Input: part model. Units: mm. Frame: model coordinates. A direction names the side the tool comes from. Coordinates: 2 decimals unless noted, no trailing zeros. Write each loop counter-clockwise with the first axis right and the second up, starting at its lowest first coordinate (ties: lowest second). Pieces come first, ordered by that corner, then holes. Notation, with made-up numbers: M 73.5,-15 L 117.5,-15 A14 cw 117.5,3 Z; hole C 34,64.5 d4. An arc over 180 degrees is marked long. Use one line per item in the form item = value.
from build123d import *

# Parameters (mm, degrees)
BOSS_EXTRUDE1_DEPTH = 60
SKETCH2_R           = 1.55
CUT_EXTRUDE1_DEPTH  = 6
SKETCH4_W           = 35
SKETCH4_H           = 30
CUT_EXTRUDE3_DEPTH  = 15
SKETCH5_R           = 1.35
CUT_EXTRUDE4_DEPTH  = 5


with BuildPart() as part:
    # Sketch1 → Boss-Extrude1 (new body)
    with BuildSketch(Plane(origin=(0, 0, 0), x_dir=(1, 0, 0), z_dir=(0, 1, 0))):
        with BuildLine():
            ThreePointArc((-42.142615011, 25), (-48.692157925, 5.483954466), (-46.647615159, -15))
            Line((-46.647615159, -15), (-41.36423576, -15))
            Line((-41.36423576, -15), (-35, -15))
            Line((-35, -15), (-35, -10))
            Line((-35, -10), (-42.848570571, -10))
            ThreePointArc((-42.848570571, -10), (-43.67673377, 5.323807579), (-39.191835885, 20))
            Line((-39.191835885, 20), (-35, 20))
            Line((-35, 20), (-35, 25))
            Line((-35, 25), (-36.20773398, 25))
            Line((-36.20773398, 25), (-42.142615011, 25))
        make_face()
    extrude(amount=BOSS_EXTRUDE1_DEPTH)

    # Sketch2 → Cut-Extrude1 (cut, through all)
    with BuildSketch(Plane(origin=(0, 0, 10), x_dir=(-1, 0, 0), z_dir=(0, 0, -1))):
        with Locations((39.997615159, 50)):
            Circle(SKETCH2_R)
        with Locations((39.997615159, 10)):
            Circle(SKETCH2_R)
    extrude(amount=-CUT_EXTRUDE1_DEPTH, mode=Mode.SUBTRACT)

    # Sketch4 → Cut-Extrude3 (cut, through all)
    with BuildSketch(Plane(origin=(-35, 0, 0), x_dir=(0, 0, -1), z_dir=(1, 0, 0))):
        with Locations((7.5, 30)):
            Rectangle(SKETCH4_W, SKETCH4_H)
    extrude(amount=-CUT_EXTRUDE3_DEPTH, mode=Mode.SUBTRACT)

    # Sketch5 → Cut-Extrude4 (cut)
    with BuildSketch(Plane(origin=(-35, 0, 0), x_dir=(0, 0, -1), z_dir=(1, 0, 0))):
        with Locations((-12, 57)):
            Circle(SKETCH5_R)
        with Locations((22, 57)):
            Circle(SKETCH5_R)
        with Locations((-12, 3)):
            Circle(SKETCH5_R)
        with Locations((22, 3)):
            Circle(SKETCH5_R)
    extrude(amount=-CUT_EXTRUDE4_DEPTH, mode=Mode.SUBTRACT)


solid = part.part
(1) Section query B-B on z = -22. Return the cut outline in (x, y).
Computed:
outline = M -43.78,0 L -35,0 L -35,1.65 L -40,1.65 L -40,4.35 L -35,4.35 L -35,15 L -43.78,15 Z; M -43.78,45 L -35,45 L -35,55.65 L -40,55.65 L -40,58.35 L -35,58.35 L -35,60 L -43.78,60 Z
(2) Set-up query: faces 4 (the flat face through (-45, 15, -7)), 5 (the flat face through (-39, 7, -25)), 6 (the cylindrical face through (-40.713, 48.625, 12.465)), 7 (the flat face through (-40, 3, -22)). Return all of +Z, -Z, +X, -X, +Y, -Y with unobstructed straight access to the full face (end or side cutting, diameter ignored); none if empty.
Computed:
face_4 = -Z, +X, -X
face_5 = -Z, +X, -X, +Y, -Y
face_6 = +Z
face_7 = +X
(3) First-contact query: pin 1 Ø4 at (x, y) = (-40, 10) entering from +Z; pin 2 Ø1.4 at (y, z) = (57, -22.5) entering from +X; pin 3 Ø1.6 at (y, z) = (57, -22) entering from -X; pin 4 Ø7 at (x, z) = (-39.5, -6) entering from +Y. Flat tips, straight axial feed; report the tip coordinate or a pass-through.
Computed:
pin_1 = 15
pin_2 = -40
pin_3 = -44.18
pin_4 = through
(4) Section query C-C on y = 10. Return the cut outline in (x, z).
Computed:
outline = M -46.65,15 A49 ccw -42.14,-25 L -35,-25 L -35,-20 L -39.19,-20 A44 cw -42.85,10 L -41.55,10 L -41.55,15 Z; M -38.45,10 L -35,10 L -35,15 L -38.45,15 Z
(5) Section query A-A on x = -37.5. Return the cut outline in (y, z).
Computed:
outline = M 0,-25 L 15,-25 L 15,-20 L 0,-20 Z; M 0,10 L 60,10 L 60,15 L 0,15 Z; M 45,-25 L 60,-25 L 60,-20 L 45,-20 Z; hole C 3,-22 d2.7; hole C 3,12 d2.7; hole C 57,-22 d2.7; hole C 57,12 d2.7
(6) Pull-direction query (Z, two-part tool) for faces 1 (the flat face through (-35, 30, 13)), 2 (the cylindrical face through (-37.465, 3.406, -23.288)), 3 (the cylindrical face through (-47.376, 29.58, 12.51)); classes: pulls with the +Z half, pulls with the -Z half, needs draft (parallel to the pull), parting line crosses it, or undercut.
Computed:
face_1 = needs draft
face_2 = undercut
face_3 = parting line crosses it
(7) Line query: probe 1 along Y at (x, z) = (-37.75, -22); probe 2 along Y at (x, z) = (-37.5, 12); probe 3 along Y at (x, z) = (-43.25, -19). Output: solid intervals per line, ascending.
Computed:
probe_1 = 0 to 1.65, 4.35 to 15, 45 to 55.65, 58.35 to 60
probe_2 = 0 to 1.65, 4.35 to 55.65, 58.35 to 60
probe_3 = 0 to 15, 45 to 60
(8) Section query D-D on z = 12. Return the cut outline in (x, y), plus the area to 3 significant figures.
Computed:
outline = M -47.51,0 L -35,0 L -35,1.65 L -40,1.65 L -40,4.35 L -35,4.35 L -35,55.65 L -40,55.65 L -40,58.35 L -35,58.35 L -35,60 L -47.51,60 Z; hole C -40,10 d3.1; hole C -40,50 d3.1
area = 708 mm^2
